Design review of the part shown in the three views and the two pictorial views. Dimensions are in mm from the part's minimum x, y and z. Round coordinates to 2 decimals unless told otherwise and drop trailing zeros. Loops run counter-clockwise (first coordinate to the right, second up) from the corner with the lowest first, then second, coordinate; pieces in that order, holes last. Notation, with made-up numbers: (62, 86.5) -> (78, 86.5) arc R29 ccw to (78, 112.5) -> close; hole circle Ø11 at (51, 84.25). An arc over 180 degrees is marked (long way). Return JSON: item names as keys, results as strings. Group by question number.
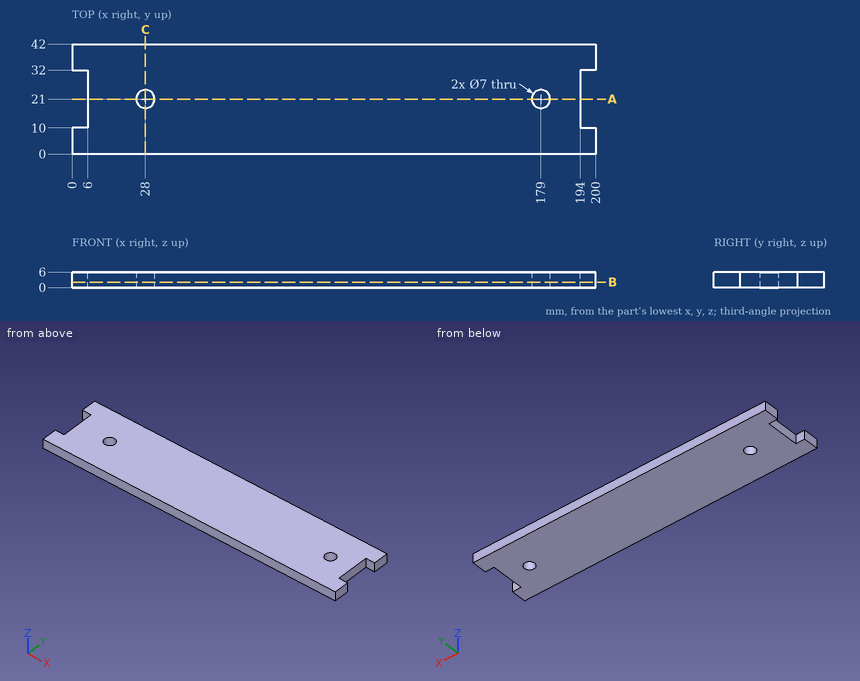
1. For P1, Ø10, axis at x = 127.5, y = 12, coming from the -Z side; P2, Ø4, axis at x = 28, y = 21, coming from the -Z side; P3, Ø3, axis at y = 20, z = 1.5, coming from the -X side, all flat-tipped, find the tip position at first contact; note any pin that passes through.
2. We need section A-A, the plane y = 21. Write out the cut boundary in (x, z).
3. Wall thickness on line 1 (Y direction, x = 28, z = 4.5); line 2 (X direction, y = 19, z = 3.4); line 3 (X direction, y = 25, z = 4.5): over which ranges is each line inside the solid? List them lowest first.
4. We need section B-B, the plane z = 2.15. Write out the cut boundary in (x, y).
5. We need section C-C, the plane x = 28. Write out the cut boundary in (y, z), then the cut area to 3 significant figures.
Check sheet entries:
{
 "1": {"P1": "stops at z = 0", "P2": "passes through", "P3": "stops at x = 6"},
 "2": {"outline": "(6, 0) -> (24.5, 0) -> (24.5, 6) -> (6, 6) -> close; (31.5, 0) -> (175.5, 0) -> (175.5, 6) -> (31.5, 6) -> close; (182.5, 0) -> (194, 0) -> (194, 6) -> (182.5, 6) -> close"},
 "3": {"line 1": "y = 0 to 17.5, 24.5 to 42", "line 2": "x = 6 to 25.13, 30.87 to 176.13, 181.87 to 194", "line 3": "x = 6 to 194"},
 "4": {"outline": "(0, 0) -> (200, 0) -> (200, 10) -> (194, 10) -> (194, 32) -> (200, 32) -> (200, 42) -> (0, 42) -> (0, 32) -> (6, 32) -> (6, 10) -> (0, 10) -> close; hole circle Ø7 at (28, 21); hole circle Ø7 at (179, 21)"},
 "5": {"outline": "(0, 0) -> (17.5, 0) -> (17.5, 6) -> (0, 6) -> close; (24.5, 0) -> (42, 0) -> (42, 6) -> (24.5, 6) -> close", "area": "210 mm²"}
}
